Source: three-view drawing plus pictorial views. Frame: mm from the lowest corner of the part. Give positions to 0.01 mm unless a question says otherwise; leave off trailing zeros. Loops run counter-clockwise (first coordinate to the right, second up) from the corner with the lowest first, then second, coordinate; pieces in that order, holes last. Notation, with made-up numbers: (-29, 47.25) -> (-18, 47.25) arc R22 ccw to (-18, 77.25) -> close; hole circle Ø3 at (57, -19.75). An arc over 180 degrees is marked (long way). One line per item, written item: value. Start each with the question number.
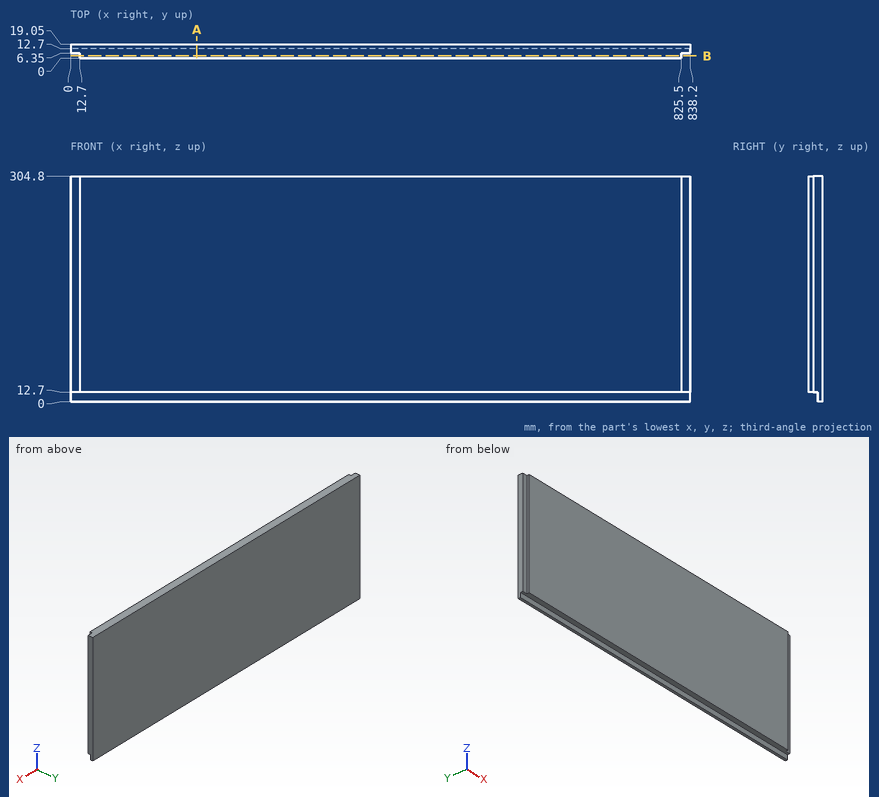
Item 1: Pin query (flat end, axial travel): pin 1 (5 mm diameter, centred on y = 2.5, z = 123.5, fed in from +X); pin 2 (10 mm diameter, centred on x = 831, z = 151, fed in from -Y); pin 3 (4 mm diameter, centred on x = 377, y = 7.5, fed in from -Z). Return the tip coordinate at first contact, or that it passes through.
Item 2: Section A-A, the plane x = 171. Output: boundary loops of the cut face in (y, z), then the cut area to 3 significant figures.
Item 3: Section B-B, the plane y = 3. Output: boundary loops of the cut face in (x, z), then the cut area to 3 significant figures.
Item 4: Ray query, line 1 along X through (y, z) = (4, 98); line 2 along Z through (x, y) = (678, 5.5). Return the intervals inside material, ascending. Write a range as [from, to].
Geometry check:
1. pin 1: stops at x = 825.5
1. pin 2: stops at y = 6.35
1. pin 3: stops at z = 12.7
2. outline: (0, 12.7) -> (12.7, 12.7) -> (12.7, 0) -> (19.05, 0) -> (19.05, 304.8) -> (0, 304.8) -> close
2. area: 5,650 mm2
3. outline: (12.7, 12.7) -> (825.5, 12.7) -> (825.5, 304.8) -> (12.7, 304.8) -> close
3. area: 237,000 mm2
4. line 1: x = [12.7, 825.5]
4. line 2: z = [12.7, 304.8]
